Geometry: final body of the model. Coordinates: model frame, mm. Face numbers are marked on the shaded views. A direction names the side the tool comes from. Give positions to 0.01 mm unless a question says otherwise; leave off trailing zeros. Write each loop counter-clockwise with the first axis right and the second up, starting at its lowest first coordinate (ties: lowest second). Pieces come first, ordered by that corner, then holes.
Q1. Reachability of the marked faces 4 and 5 from +Z, -Z, +X, -X, +Y, -Y: full face, straight path, thin tool, end or side. Return the list, or none.
Q2. Section A-A (x = 6.25). State how many separate pieces and enclosed holes the cut face has, plus the area to 3 significant figures.
Q3. Mould query, pull axis Z, two halves, no side actions, for the marked faces 1, 2 and 3. Classes: +Z half, -Z half, draft (parallel to the pull), parting line (faces both ways), or undercut.
Q4. Line query: line 1 (Y direction, x = 15, z = -13); line 2 (Z direction, x = 13.5, y = -30); line 3 (Y direction, x = 6.75, z = 9). Output: solid intervals per line, ascending.
Q5. Pin query (flat end, axial travel): pin 1 Ø2 at (y, z) = (17, 0) entering from -X; pin 2 Ø4 at (y, z) = (-28.5, -8) entering from -X; pin 3 Ø2.5 at (y, z) = (-30, -13) entering from -X. Return the tip coordinate at first contact, or that it passes through.
Q6. Section B-B (z = 16.5). Return the cut outline in (x, y).
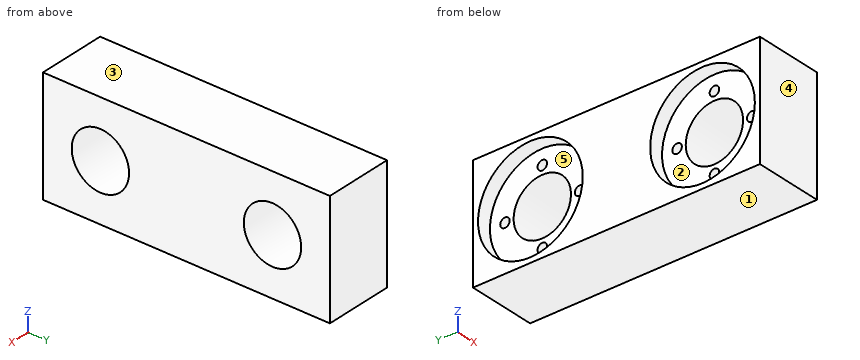
from build123d import *

# Parameters (mm, degrees)
F0_W     = 100
F0_H     = 40
F0_R     = 10
F1_DEPTH = 24
F2_R     = 18.25
F2_R_2   = 10
F3_DEPTH = 5
F5_D     = 3.3
F5_DEPTH = 14.1
F5_TIP   = 0.9914200214


with BuildPart() as f1:
    # F0 (on Right) → F1 (new body)
    with BuildSketch(Plane.YZ):
        Rectangle(F0_W, F0_H)
        with Locations((-30, 0)):
            Circle(F0_R, mode=Mode.SUBTRACT)
        with Locations((30, 0)):
            Circle(F0_R, mode=Mode.SUBTRACT)
    extrude(amount=F1_DEPTH)

    # F2 (on face) → F3 (cut)
    with BuildSketch(Plane(origin=(0, 0, 0), x_dir=(0, -1, 0), z_dir=(-1, 0, 0))):
        with Locations((-30, 0)):
            Circle(F2_R)
        with Locations((-30, 0)):
            Circle(F2_R_2, mode=Mode.SUBTRACT)
        with Locations((30, 0)):
            Circle(F2_R)
        with Locations((30, 0)):
            Circle(F2_R_2, mode=Mode.SUBTRACT)
    extrude(amount=-F3_DEPTH, mode=Mode.SUBTRACT)

    # F5
    with Locations(Plane(origin=(5, 0, 0), x_dir=(0, -1, 0), z_dir=(-1, 0, 0))):
        with Locations((-43, 0), (-30, 13), (-17, 0), (-30, -13), (17, 0), (30, 13), (43, 0), (30, -13)):
            Hole(F5_D / 2, depth=F5_DEPTH)
            with Locations((0, 0, -(F5_DEPTH + F5_TIP / 2))):  # 118° drill point
                Cone(0, F5_D / 2, F5_TIP, mode=Mode.SUBTRACT)


solid = f1.part
Computed:
1. face 4: +Z, -Z, +X, -X, -Y
1. face 5: -X
2. separate pieces: 1
2. enclosed holes: 10
2. area: 3,300 mm2
3. face 1: -Z half
3. face 2: undercut
3. face 3: +Z half
4. line 1: y = -50 to -31.65, -28.35 to 28.35, 31.65 to 50
4. line 2: z = -20 to -14.65, -11.35 to -10, 10 to 11.35, 14.65 to 20
4. line 3: y = -50 to -34.36, -25.64 to 25.64, 34.36 to 50
5. pin 1: stops at x = 19.49
5. pin 2: stops at x = 5
5. pin 3: stops at x = 19.34
6. outline: (0, -50) - (24, -50) - (24, 50) - (0, 50) - (0, 37.8) - (5, 37.8) - (5, 22.2) - (0, 22.2) - (0, -22.2) - (5, -22.2) - (5, -37.8) - (0, -37.8) - close
